The listing builds one solid part. Answer for the finished solid, in the listing's coordinates (mm). A direction names the side the tool comes from. Round coordinates to 2 decimals unless told otherwise and drop trailing zeros. Use a Markdown table: item, result. Add a question column.
Q1. Given pin 1 Ø6 at (x, z) = (316.5, 10.5) entering from -Y; pin 2 Ø1 at (x, z) = (344.5, -19) entering from +Y; pin 3 Ø3 at (x, z) = (341, 9.5) entering from +Y; pin 4 Ø1.8 at (x, z) = (285.5, 11.5) entering from -Y, each flat-ended and moving along its own axis, determine where each tip first touches the part or whether it passes through.
Q2. Which of the six approach directions +Z, -Z, +X, -X, +Y, -Y give full straight-line access (tool end or side, diameter ignored) to faces 1 (the flat face through (232, -20, 0)), 2 (the flat face through (231.71, -0.62, 0.44))?
Q3. Consider line 1 (Z direction, x = 458.5, y = -10); line 2 (Y direction, x = 431, z = 17); line 3 (Y direction, x = 459, z = 10). Determine where each line is inside the solid, lowest interval first.
Q4. Section A-A on x = 140.5 is taken. Give the number of separate pieces and of enclosed holes in the cut face, then the cut area to 3 significant figures.
from build123d import *

# Parameters (mm, degrees)
SKETCH1_R           = 2.1
BOSS_EXTRUDE1_DEPTH = 470
SKETCH10_R          = 2.1
BOSS_EXTRUDE4_DEPTH = 15
BOSS_EXTRUDE5_START = -15
SKETCH11_R          = 2.1
BOSS_EXTRUDE5_DEPTH = 15
TAPPED_HOLE3_D      = 4.2
TAPPED_HOLE3_DEPTH  = 15
TAPPED_HOLE4_D      = 4.2


with BuildPart() as part:
    # Sketch1 → Boss-Extrude1 (new body)
    with BuildSketch(Plane(origin=(0, 0, 0), x_dir=(0, 0, -1), z_dir=(1, 0, 0))):
        with BuildLine():
            Line((-13, 18), (-13, 20))
            Line((-13, 20), (-19, 20))
            ThreePointArc((-19, 20), (-19.707106781, 19.707106781), (-20, 19))
            Line((-20, 19), (-20, 13))
            Line((-20, 13), (-18, 13))
            Line((-18, 13), (-18, 16))
            Line((-18, 16), (-17.060660172, 16))
            Line((-17.060660172, 16), (-14, 12.939339828))
            Line((-14, 12.939339828), (-14, 7.060660172))
            Line((-14, 7.060660172), (-17.060660172, 4))
            Line((-17.060660172, 4), (-18, 4))
            Line((-18, 4), (-18, 7))
            Line((-18, 7), (-20, 7))
            Line((-20, 7), (-20, -7))
            Line((-20, -7), (-18, -7))
            Line((-18, -7), (-18, -4))
            Line((-18, -4), (-17.060660172, -4))
            Line((-17.060660172, -4), (-14, -7.060660172))
            Line((-14, -7.060660172), (-14, -12.939339828))
            Line((-14, -12.939339828), (-17.060660172, -16))
            Line((-17.060660172, -16), (-18, -16))
            Line((-18, -16), (-18, -13))
            Line((-18, -13), (-20, -13))
            Line((-20, -13), (-20, -19))
            ThreePointArc((-20, -19), (-19.707106781, -19.707106781), (-19, -20))
            Line((-19, -20), (-13, -20))
            Line((-13, -20), (-13, -18))
            Line((-13, -18), (-16, -18))
            Line((-16, -18), (-16, -17.060660172))
            Line((-16, -17.060660172), (-12.939339828, -14))
            Line((-12.939339828, -14), (-7.060660172, -14))
            Line((-7.060660172, -14), (-4, -17.060660172))
            Line((-4, -17.060660172), (-4, -18))
            Line((-4, -18), (-7, -18))
            Line((-7, -18), (-7, -20))
            Line((-7, -20), (7, -20))
            Line((7, -20), (7, -18))
            Line((7, -18), (4, -18))
            Line((4, -18), (4, -17.060660172))
            Line((4, -17.060660172), (7.060660172, -14))
            Line((7.060660172, -14), (12.939339828, -14))
            Line((12.939339828, -14), (16, -17.060660172))
            Line((16, -17.060660172), (16, -18))
            Line((16, -18), (13, -18))
            Line((13, -18), (13, -20))
            Line((13, -20), (19, -20))
            ThreePointArc((19, -20), (19.707106781, -19.707106781), (20, -19))
            Line((20, -19), (20, -13))
            Line((20, -13), (18, -13))
            Line((18, -13), (18, -16))
            Line((18, -16), (17.060660172, -16))
            Line((17.060660172, -16), (14, -12.939339828))
            Line((14, -12.939339828), (14, -7.060660172))
            Line((14, -7.060660172), (17.060660172, -4))
            Line((17.060660172, -4), (18, -4))
            Line((18, -4), (18, -7))
            Line((18, -7), (20, -7))
            Line((20, -7), (20, -1))
            ThreePointArc((20, -1), (19.707106781, -0.292893219), (19, 0))
            Line((19, 0), (13, 0))
            Line((13, 0), (13, -2))
            Line((13, -2), (16, -2))
            Line((16, -2), (16, -2.939339828))
            Line((16, -2.939339828), (12.939339828, -6))
            Line((12.939339828, -6), (7.060660172, -6))
            Line((7.060660172, -6), (4, -2.939339828))
            Line((4, -2.939339828), (4, -2))
            Line((4, -2), (7, -2))
            Line((7, -2), (7, 0))
            Line((7, 0), (0.3, 0))
            ThreePointArc((0.3, 0), (0.087867966, 0.087867966), (0, 0.3))
            Line((0, 0.3), (0, 7))
            Line((0, 7), (-2, 7))
            Line((-2, 7), (-2, 4))
            Line((-2, 4), (-2.939339828, 4))
            Line((-2.939339828, 4), (-6, 7.060660172))
            Line((-6, 7.060660172), (-6, 12.939339828))
            Line((-6, 12.939339828), (-2.939339828, 16))
            Line((-2.939339828, 16), (-2, 16))
            Line((-2, 16), (-2, 13))
            Line((-2, 13), (0, 13))
            Line((0, 13), (0, 19))
            ThreePointArc((0, 19), (-0.292893219, 19.707106781), (-1, 20))
            Line((-1, 20), (-7, 20))
            Line((-7, 20), (-7, 18))
            Line((-7, 18), (-4, 18))
            Line((-4, 18), (-4, 17.060660172))
            Line((-4, 17.060660172), (-7.060660172, 14))
            Line((-7.060660172, 14), (-12.939339828, 14))
            Line((-12.939339828, 14), (-16, 17.060660172))
            Line((-16, 17.060660172), (-16, 18))
            Line((-16, 18), (-13, 18))
        make_face()
        with Locations(Location((10, -10, 0), (0, 0, 180))):
            Circle(SKETCH1_R, mode=Mode.SUBTRACT)
        with Locations(Location((-10, 10, 0), (0, 0, 180))):
            Circle(SKETCH1_R, mode=Mode.SUBTRACT)
        Polygon((6, -7.060660172), (-7.060660172, 6), (-12.939339828, 6), (-16.439339828, 2.5), (-18, 2.5), (-18, -2.5), (-16.439339828, -2.5), (-12.5, -6.439339828), (-12.5, -12.5), (-6.439339828, -12.5), (-2.5, -16.439339828), (-2.5, -18), (2.5, -18), (2.5, -16.439339828), (6, -12.939339828), align=None, mode=Mode.SUBTRACT)
    extrude(amount=BOSS_EXTRUDE1_DEPTH)

    # Sketch10 → Boss-Extrude4 (add)
    with BuildSketch(Plane(origin=(0, 0, 0), x_dir=(0, 0, -1), z_dir=(1, 0, 0))):
        with Locations(Location((10, -10, 0), (0, 0, 180))):
            Circle(SKETCH10_R)
        with Locations(Location((-10, 10, 0), (0, 0, 180))):
            Circle(SKETCH10_R)
    extrude(amount=BOSS_EXTRUDE4_DEPTH)

    # Sketch11 → Boss-Extrude5 (add)
    with BuildSketch(Plane(origin=(470, 0, 0), x_dir=(0, 0, -1), z_dir=(1, 0, 0)).offset(BOSS_EXTRUDE5_START)):
        with Locations(Location((10, -10, 0), (0, 0, 180))):
            Circle(SKETCH11_R)
        with Locations(Location((-10, 10, 0), (0, 0, 180))):
            Circle(SKETCH11_R)
    extrude(amount=BOSS_EXTRUDE5_DEPTH)

    # Tapped Hole3
    with Locations(Plane(origin=(0, 0, 42.543082138), x_dir=(0, 0, -1), z_dir=(-1, 0, 0))):
        with Locations((52.543082138, 10), (32.543082138, -10)):
            Hole(TAPPED_HOLE3_D / 2, depth=TAPPED_HOLE3_DEPTH)

    # Tapped Hole4 (through all)
    with Locations(Plane(origin=(470, 0, -41.216277394), x_dir=(0, 0, 1), z_dir=(1, 0, 0))):
        with Locations((51.216277394, -10), (31.216277394, 10)):
            Hole(TAPPED_HOLE4_D / 2)


solid = part.part
Checked values:
| question | item | result |
|---|---|---|
| 1 | pin 1 | stops at y = -20 |
| 1 | pin 2 | stops at y = 0 |
| 1 | pin 3 | stops at y = 14 |
| 1 | pin 4 | stops at y = -14 |
| 2 | face 1 | +Z, -Z, +X, -X, -Y |
| 2 | face 2 | +X, -X |
| 3 | line 1 | z = -14 to -12.1, -7.9 to -6, 12.5 to 14 |
| 3 | line 2 | y = -20 to -15.94, -4.06 to -2.5, 2.5 to 4.06, 15.94 to 20 |
| 3 | line 3 | y = -14 to -12.5, 6 to 7.9, 12.1 to 14 |
| 4 | separate pieces | 1 |
| 4 | enclosed holes | 3 |
| 4 | area | 423 mm2 |
